```python
from build123d import *

# Parameters (mm, degrees)
F0_W     = 26
F0_H     = 26
F0_W_2   = 16
F0_H_2   = 16
F1_DEPTH = 3
F3_DEPTH = 22.5
F2_W     = 16
F2_H     = 1
F4_DEPTH = 5
F5_W     = 6
F5_H     = 1
F6_DEPTH = 3.5


with BuildPart() as f1:
    # F0 (on Top) → F1 (new body)
    with BuildSketch(Plane.XY):
        Rectangle(F0_W, F0_H)
        Rectangle(F0_W_2, F0_H_2, mode=Mode.SUBTRACT)
    extrude(amount=F1_DEPTH)

    # F2 (on face) → F3 (cut)
    with BuildSketch(Plane.XZ.offset(13)):
        Polygon((-8, 2), (-9.5, 2), (-9.5, 1), (9.5, 1), (9.5, 2), (8, 2), align=None)
    extrude(amount=-F3_DEPTH, mode=Mode.SUBTRACT)

    # F2 (on face) → F4 (cut, through all)
    with BuildSketch(Plane.XZ.offset(13)):
        with Locations((0, 2.5)):
            Rectangle(F2_W, F2_H)
    extrude(amount=-F4_DEPTH, mode=Mode.SUBTRACT)

    # F5 (on face) → F6 (cut, through all)
    with BuildSketch(Plane(origin=(0, 13, 0), x_dir=(-1, 0, 0), z_dir=(0, 1, 0))):
        with Locations((0, 1.5)):
            Rectangle(F5_W, F5_H)
    extrude(amount=-F6_DEPTH, mode=Mode.SUBTRACT)


solid = f1.part
```
Check sheet for the modelled part. Datum: model origin and axes. Units: mm. A direction names the side the tool comes from. Coordinates: 2 decimals unless noted, no trailing zeros. Order: outer loops, then holes, each group sorted by start corner. A loop starts at its lowest first (then second) coordinate and runs counter-clockwise, first axis right, second up. Notation, with made-up numbers: (77, 8) -> (109, 8) arc R19 ccw to (109, 27) -> close; hole circle Ø3 at (-36.75, 52). An arc over 180 degrees is marked (long way). Write each question's results on one line, items separated by ' | '. Start each with the question number.
1) Section check D-D (y = 10.75). Enter the section's corners in (x, z).
2) Depth check by flat-ended pin: pin 1 (0.8 mm diameter, centred on x = -7.5, z = 1.5, fed in from -Y); pin 2 (1 mm diameter, centred on x = -7, y = -3, fed in from -Z). Enter the tip coordinate at first touch or a pass-through.
3) Draft check along Y on faces 6 (the face through (-8, -0.1, 0.5)), 7 (the face through (9.5, -1.9, 1.5)), 8 (the face through (-0.1, 8, 0.5)), 9 (the face through (-0.2, -13, 0.8)). Enter one of: pulls with the +Y half, pulls with the -Y half, needs draft (parallel to the pull), parting line crosses it, or undercut.
4) Set-up check for faces 1 (the face through (3, 11.3, 1.5)), 2 (the face through (-0.1, -8, 0.5)), 3 (the face through (-8, -2.6, 2.5)), 4 (the face through (0, -9, 1)), 5 (the face through (-0.1, 8, 2.5)): record each of +Z, -Z, +X, -X, +Y, -Y from which the full face is reachable in a straight line by a thin tool's end or side.
5) Section check C-C (x = -2.5). Enter the section's corners in (y, z), and give its area (3 significant figures).
6) Section check A-A (z = 1.45). Enter the section's corners in (x, y).
7) Section check B-B (y = -7.25). Enter the section's corners in (x, z), and give its area (3 significant figures).
8) Material ranges on line 1 along Z through (x, y) = (-8.5, 4.5); line 2 along X through (y, z) = (-2.75, 0.9); line 3 along X through (y, z) = (7, 1.05), recorded low to high.
Checked values:
1) outline: (-13, 0) -> (13, 0) -> (13, 3) -> (-13, 3) -> close; hole (-3, 1) -> (3, 1) -> (3, 2) -> (-3, 2) -> close
2) pin 1: y = 9.5 | pin 2: through
3) face 6: undercut | face 7: needs draft | face 8: undercut | face 9: pulls with the -Y half
4) face 1: +Y, -Y | face 2: +Z, -Z | face 3: +Z, -Y | face 4: -Y | face 5: +Z, -Z, -Y
5) outline: (-13, 0) -> (-8, 0) -> (-8, 1) -> (-13, 1) -> close; (8, 0) -> (13, 0) -> (13, 1) -> (8, 1) -> close; (8, 2) -> (13, 2) -> (13, 3) -> (8, 3) -> close | area: 15.0 mm²
6) outline: (-13, -13) -> (-9.5, -13) -> (-9.5, 9.5) -> (-3, 9.5) -> (-3, 13) -> (-13, 13) -> close; (3, 9.5) -> (9.5, 9.5) -> (9.5, -13) -> (13, -13) -> (13, 13) -> (3, 13) -> close
7) outline: (-13, 0) -> (-8, 0) -> (-8, 1) -> (-9.5, 1) -> (-9.5, 2) -> (-8, 2) -> (-8, 3) -> (-13, 3) -> close; (8, 0) -> (13, 0) -> (13, 3) -> (8, 3) -> (8, 2) -> (9.5, 2) -> (9.5, 1) -> (8, 1) -> close | area: 27.0 mm²
8) line 1: 0 to 1, 2 to 3 | line 2: -13 to -8, 8 to 13 | line 3: -13 to -9.5, 9.5 to 13
